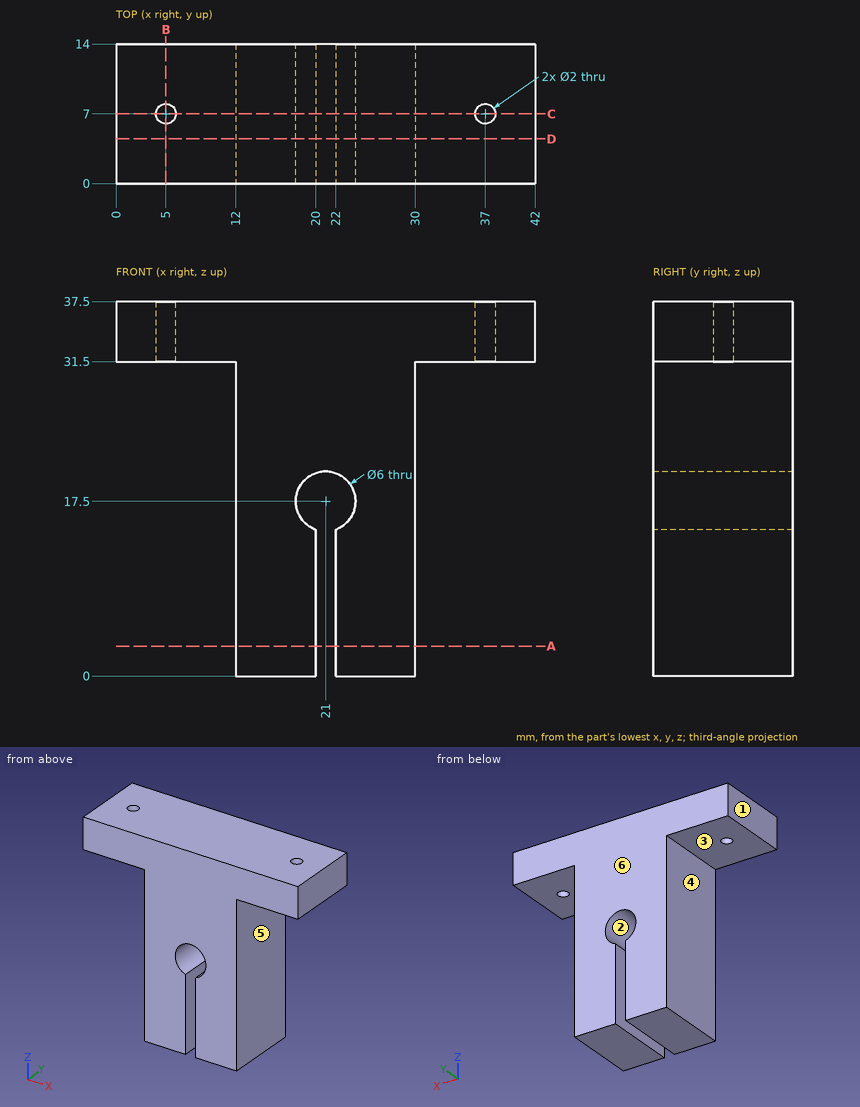
Job drawing, mm, ordinate dimensions from the low corner. One solid piece. A direction names the side the tool comes from. Coordinates: 2 decimals unless noted, no trailing zeros. Write each loop counter-clockwise with the first axis right and the second up, starting at its lowest first coordinate (ties: lowest second). Pieces come first, ordered by that corner, then holes.
Item 1: Slice it at A-A (z = 3). Write the cut outline in (x, y), and give its area (3 significant figures).
Item 2: Probe line 1 (X direction, y = 5.25, z = 8); line 2 (Y direction, x = 37, z = 35); line 3 (X direction, y = 10, z = 17.5). List the from-to ranges inside material, lowest first.
Item 3: Slice it at C-C (y = 7). Write the cut outline in (x, z).
Item 4: Slice it at B-B (x = 5). Write the cut outline in (y, z), and give its area (3 significant figures).
Item 5: Pin check, flat tips, straight feed: pin 1 (1.5 mm diameter, centred on x = 16.5, y = 7.5, fed in from -Z); pin 2 (7 mm diameter, centred on y = 4, z = 9.5, fed in from -X); pin 3 (7 mm diameter, centred on y = 6, z = 12, fed in from +X). Stop position of each tip, or through.
Item 6: Which spindle directions (+Z, -Z, +X, -X, +Y, -Y) get a long thin tool onto all of the face, cutting with end or side? Do the marked faces 4, 5 and 6. Say none if no direction does.
Item 7: Slice it at D-D (y = 4.5). Write the cut outline in (x, z), and give its area (3 significant figures).
Item 8: Mould opens along Z. For the marked faces 1, 2 and 3 say: released by +Z, released by -Z, zero draft, split by the parting line, or undercut.
Results found:
1. outline: (12, 0) - (20, 0) - (20, 14) - (12, 14) - close; (22, 0) - (30, 0) - (30, 14) - (22, 14) - close
1. area: 224 mm2
2. line 1: x = 12 to 20, 22 to 30
2. line 2: y = 0 to 6, 8 to 14
2. line 3: x = 12 to 18, 24 to 30
3. outline: (0, 31.5) - (4, 31.5) - (4, 37.5) - (0, 37.5) - close; (6, 31.5) - (12, 31.5) - (12, 0) - (20, 0) - (20, 14.67) arc R3 cw (long way) to (22, 14.67) - (22, 0) - (30, 0) - (30, 31.5) - (36, 31.5) - (36, 37.5) - (6, 37.5) - close; (38, 31.5) - (42, 31.5) - (42, 37.5) - (38, 37.5) - close
4. outline: (0, 31.5) - (6, 31.5) - (6, 37.5) - (0, 37.5) - close; (8, 31.5) - (14, 31.5) - (14, 37.5) - (8, 37.5) - close
4. area: 72.0 mm2
5. pin 1: stops at z = 0
5. pin 2: stops at x = 12
5. pin 3: stops at x = 30
6. face 4: -Z, -X, +Y, -Y
6. face 5: -Z, +X, +Y, -Y
6. face 6: +Z, -Z, +X, -X, +Y
7. outline: (0, 31.5) - (12, 31.5) - (12, 0) - (20, 0) - (20, 14.67) arc R3 cw (long way) to (22, 14.67) - (22, 0) - (30, 0) - (30, 31.5) - (42, 31.5) - (42, 37.5) - (0, 37.5) - close
7. area: 762 mm2
8. face 1: zero draft
8. face 2: undercut
8. face 3: released by -Z
